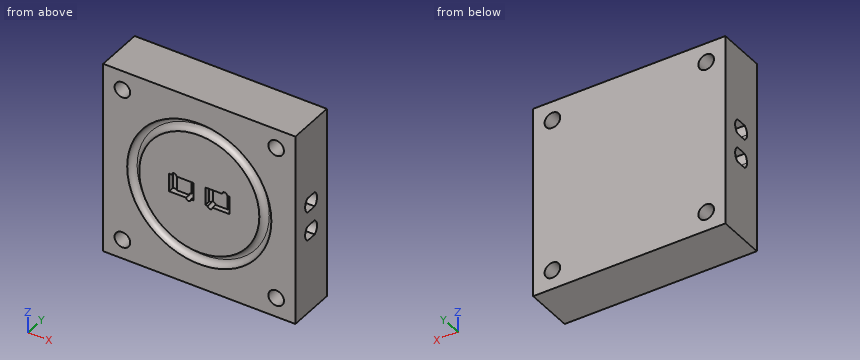
from build123d import *

# Parameters (mm, degrees)
F1_W      = 80
F1_H      = 80
F2_DEPTH  = 20
F4_R      = 3.25
F5_DEPTH  = 20.001
F4_R_2    = 30
F4_R_3    = 25
F6_DEPTH  = 2.5
F7_R      = 2.49999
F4_W      = 2
F4_H      = 3.75
F9_DEPTH  = 2.5
F10_DEPTH = 10
F12_DEPTH = 80.001
F13_DEPTH = 80.0010001
F14_DEPTH = 2


# Not quite as in the source:
# - two fillets or chamfers of one size are made in one step
# - a fillet or chamfer is up to 0.001 mm smaller than in the source, because OpenCascade refuses the exact size


with BuildPart() as f2:
    # F1 (on Front) → F2 (new body)
    with BuildSketch(Plane.XZ):
        with Locations((40, 40)):
            Rectangle(F1_W, F1_H)
    extrude(amount=F2_DEPTH)

    # F4 (on face) → F5 (cut, through all)
    with BuildSketch(Plane.XZ.offset(20)):
        with Locations((72, 8)):
            Circle(F4_R)
        with Locations((8, 8)):
            Circle(F4_R)
        with Locations((8, 72)):
            Circle(F4_R)
        with Locations((72, 72)):
            Circle(F4_R)
    extrude(amount=-F5_DEPTH, mode=Mode.SUBTRACT)

    # F4 (on face) → F6 (cut)
    with BuildSketch(Plane.XZ.offset(20)):
        with Locations((40, 40)):
            Circle(F4_R_2)
        with Locations((40, 40)):
            Circle(F4_R_3, mode=Mode.SUBTRACT)
    extrude(amount=-F6_DEPTH, mode=Mode.SUBTRACT)

    # F7 (radius 2.5 in the source; OpenCascade refuses exactly that, so slightly less here)
    f7_edges = [f2.edges().sort_by_distance(p)[0] for p in [
        (15, -17.5, 40),
        (10, -17.5, 40),
    ]]
    fillet(f7_edges, radius=F7_R)

    # F4 (on face) → F9 (cut)
    with BuildSketch(Plane.XZ.offset(20)):
        with BuildLine():
            Line((28.5, 43.75), (27.5, 43.75))
            Line((27.5, 43.75), (27.5, 40))
            Line((27.5, 40), (29.5, 40))
            Line((29.5, 40), (29.5, 42.75))
            ThreePointArc((29.5, 42.75), (28.7928932188, 43.0428932188), (28.5, 43.75))
        make_face()
        with Locations((28.5, 38.125)):
            Rectangle(F4_W, F4_H)
        with BuildLine():
            ThreePointArc((30.5, 43.75), (29.5, 44.75), (28.5, 43.75))
            Line((28.5, 43.75), (29.5, 43.75))
            Line((29.5, 43.75), (30.5, 43.75))
        make_face()
        with BuildLine():
            Line((52.5, 40), (52.5, 43.75))
            Line((52.5, 43.75), (51.5, 43.75))
            ThreePointArc((51.5, 43.75), (51.2071067812, 43.0428932188), (50.5, 42.75))
            Line((50.5, 42.75), (50.5, 40))
            Line((50.5, 40), (52.5, 40))
        make_face()
        with BuildLine():
            Line((37.5, 36.25), (37.5, 40))
            Line((37.5, 40), (35.5, 40))
            Line((35.5, 40), (35.5, 37.25))
            ThreePointArc((35.5, 37.25), (36.2071067812, 36.9571067812), (36.5, 36.25))
            Line((36.5, 36.25), (37.5, 36.25))
        make_face()
        with Locations((36.5, 41.875)):
            Rectangle(F4_W, F4_H)
        with Locations((43.5, 41.875)):
            Rectangle(F4_W, F4_H)
        with BuildLine():
            Line((44.5, 40), (42.5, 40))
            Line((42.5, 40), (42.5, 36.25))
            Line((42.5, 36.25), (43.5, 36.25))
            ThreePointArc((43.5, 36.25), (43.7928932188, 36.9571067812), (44.5, 37.25))
            Line((44.5, 37.25), (44.5, 40))
        make_face()
        with Locations((51.5, 38.125)):
            Rectangle(F4_W, F4_H)
        with BuildLine():
            Line((50.5, 43.75), (51.5, 43.75))
            ThreePointArc((51.5, 43.75), (50.5, 44.75), (49.5, 43.75))
            Line((49.5, 43.75), (50.5, 43.75))
        make_face()
        with BuildLine():
            ThreePointArc((36.5, 36.25), (36.2071067812, 36.9571067812), (35.5, 37.25))
            Line((35.5, 37.25), (35.5, 36.25))
            Line((35.5, 36.25), (36.5, 36.25))
        make_face()
        with BuildLine():
            Line((44.5, 36.25), (44.5, 37.25))
            ThreePointArc((44.5, 37.25), (43.7928932188, 36.9571067812), (43.5, 36.25))
            Line((43.5, 36.25), (44.5, 36.25))
        make_face()
    extrude(amount=-F9_DEPTH, mode=Mode.SUBTRACT)

    # F4 (on face) → F10 (cut)
    with BuildSketch(Plane.XZ.offset(20)):
        with BuildLine():
            ThreePointArc((30.5, 43.75), (29.5, 44.75), (28.5, 43.75))
            Line((28.5, 43.75), (29.5, 43.75))
            Line((29.5, 43.75), (30.5, 43.75))
        make_face()
        with BuildLine():
            Line((29.5, 43.75), (28.5, 43.75))
            ThreePointArc((28.5, 43.75), (28.7928932188, 43.0428932188), (29.5, 42.75))
            Line((29.5, 42.75), (29.5, 43.75))
        make_face()
        with BuildLine():
            Line((30.5, 43.75), (29.5, 43.75))
            Line((29.5, 43.75), (29.5, 42.75))
            ThreePointArc((29.5, 42.75), (30.2071067812, 43.0428932188), (30.5, 43.75))
        make_face()
        with BuildLine():
            Line((35.5, 36.25), (35.5, 37.25))
            ThreePointArc((35.5, 37.25), (34.7928932188, 36.9571067812), (34.5, 36.25))
            Line((34.5, 36.25), (35.5, 36.25))
        make_face()
        with BuildLine():
            ThreePointArc((36.5, 36.25), (36.2071067812, 36.9571067812), (35.5, 37.25))
            Line((35.5, 37.25), (35.5, 36.25))
            Line((35.5, 36.25), (36.5, 36.25))
        make_face()
        with BuildLine():
            ThreePointArc((34.5, 36.25), (35.5, 35.25), (36.5, 36.25))
            Line((36.5, 36.25), (35.5, 36.25))
            Line((35.5, 36.25), (34.5, 36.25))
        make_face()
        with BuildLine():
            Line((44.5, 36.25), (44.5, 37.25))
            ThreePointArc((44.5, 37.25), (43.7928932188, 36.9571067812), (43.5, 36.25))
            Line((43.5, 36.25), (44.5, 36.25))
        make_face()
        with BuildLine():
            ThreePointArc((45.5, 36.25), (45.2071067812, 36.9571067812), (44.5, 37.25))
            Line((44.5, 37.25), (44.5, 36.25))
            Line((44.5, 36.25), (45.5, 36.25))
        make_face()
        with BuildLine():
            Line((44.5, 36.25), (43.5, 36.25))
            ThreePointArc((43.5, 36.25), (44.5, 35.25), (45.5, 36.25))
            Line((45.5, 36.25), (44.5, 36.25))
        make_face()
        with BuildLine():
            Line((50.5, 43.75), (51.5, 43.75))
            ThreePointArc((51.5, 43.75), (50.5, 44.75), (49.5, 43.75))
            Line((49.5, 43.75), (50.5, 43.75))
        make_face()
        with BuildLine():
            Line((50.5, 42.75), (50.5, 43.75))
            Line((50.5, 43.75), (49.5, 43.75))
            ThreePointArc((49.5, 43.75), (49.7928932188, 43.0428932188), (50.5, 42.75))
        make_face()
        with BuildLine():
            ThreePointArc((50.5, 42.75), (51.2071067812, 43.0428932188), (51.5, 43.75))
            Line((51.5, 43.75), (50.5, 43.75))
            Line((50.5, 43.75), (50.5, 42.75))
        make_face()
    extrude(amount=-F10_DEPTH, mode=Mode.SUBTRACT)

    # F11 (on face) → F12 (cut, through all)
    with BuildSketch(Plane(origin=(0, 0, 0), x_dir=(0, -1, 0), z_dir=(-1, 0, 0))):
        with BuildLine():
            ThreePointArc((12.2666053913, 42.95), (13.3950773546, 44.293116947), (13.8, 46))
            ThreePointArc((13.8, 46), (13.3950773546, 47.706883053), (12.2666053913, 49.05))
            Line((12.2666053913, 49.05), (7.7333946087, 49.05))
            ThreePointArc((7.7333946087, 49.05), (6.2, 46), (7.7333946087, 42.95))
            Line((7.7333946087, 42.95), (12.2666053913, 42.95))
        make_face()
    extrude(amount=-F12_DEPTH, mode=Mode.SUBTRACT)

    # F11 (on face) → F13 (cut, through all)
    with BuildSketch(Plane(origin=(0, 0, 0), x_dir=(0, -1, 0), z_dir=(-1, 0, 0))):
        with BuildLine():
            ThreePointArc((12.2666053913, 42.95), (13.3950773546, 44.293116947), (13.8, 46))
            ThreePointArc((13.8, 46), (13.3950773546, 47.706883053), (12.2666053913, 49.05))
            Line((12.2666053913, 49.05), (7.7333946087, 49.05))
            ThreePointArc((7.7333946087, 49.05), (6.2, 46), (7.7333946087, 42.95))
            Line((7.7333946087, 42.95), (12.2666053913, 42.95))
        make_face()
        with BuildLine():
            ThreePointArc((12.2666053913, 30.95), (13.3950773546, 32.293116947), (13.8, 34))
            ThreePointArc((13.8, 34), (13.3950773546, 35.706883053), (12.2666053913, 37.05))
            Line((12.2666053913, 37.05), (7.7333946087, 37.05))
            ThreePointArc((7.7333946087, 37.05), (6.2, 34), (7.7333946087, 30.95))
            Line((7.7333946087, 30.95), (12.2666053913, 30.95))
        make_face()
    extrude(amount=-F13_DEPTH, mode=Mode.SUBTRACT)

    # F4 (on face) → F14 (cut)
    with BuildSketch(Plane.XZ.offset(20)):
        with BuildLine():
            Line((29.5, 42.75), (29.5, 40))
            Line((29.5, 40), (35.5, 40))
            Line((35.5, 40), (35.5, 43.75))
            Line((35.5, 43.75), (30.5, 43.75))
            ThreePointArc((30.5, 43.75), (30.2071067812, 43.0428932188), (29.5, 42.75))
        make_face()
        with BuildLine():
            Line((35.5, 40), (29.5, 40))
            Line((29.5, 40), (29.5, 36.25))
            Line((29.5, 36.25), (34.5, 36.25))
            ThreePointArc((34.5, 36.25), (34.7928932188, 36.9571067812), (35.5, 37.25))
            Line((35.5, 37.25), (35.5, 40))
        make_face()
        with BuildLine():
            Line((44.5, 43.75), (44.5, 40))
            Line((44.5, 40), (50.5, 40))
            Line((50.5, 40), (50.5, 42.75))
            ThreePointArc((50.5, 42.75), (49.7928932188, 43.0428932188), (49.5, 43.75))
            Line((49.5, 43.75), (44.5, 43.75))
        make_face()
        with BuildLine():
            Line((50.5, 40), (44.5, 40))
            Line((44.5, 40), (44.5, 37.25))
            ThreePointArc((44.5, 37.25), (45.2071067812, 36.9571067812), (45.5, 36.25))
            Line((45.5, 36.25), (50.5, 36.25))
            Line((50.5, 36.25), (50.5, 40))
        make_face()
    extrude(amount=-F14_DEPTH, mode=Mode.SUBTRACT)


solid = f2.part
Part model, mm, in its own coordinate system. Give positions to 0.01 mm unless a question says otherwise; leave off trailing zeros. Loops run counter-clockwise (first coordinate to the right, second up) from the corner with the lowest first, then second, coordinate; pieces in that order, holes last. Notation, with made-up numbers: M -8.5,-26 L -4.5,-26 A15 cw -4.5,-10 Z; hole C -36,82.5 d10. An arc over 180 degrees is marked long. Put each result on its own line as item: value. Start each with the question number.
1) Probe probe 1 along Z at (x, y) = (72, -8.5); probe 2 along Z at (x, y) = (32, -9.5); probe 3 along X at (y, z) = (-17.25, 43.75). List the from-to ranges inside material, lowest first.
2) Saw through at C-C (y = -4.75). List the corners of the cut face in (x, z).
3) Saw through at B-B (z = 72). List the corners of the cut face in (x, y), then the cut area to 3 significant figures.
4) Flat gauge pin, fed straight in: pin 1 (0.6 mm diameter, centred on x = 51, z = 39, fed in from -Y). Where does the tip first touch, or does it go through?
5) Saw through at A-A (x = 8). List the corners of the cut face in (y, z), then the cut area to 3 significant figures.
6) Saw through at D-D (x = 33). State how many separate pieces and enclosed holes the cut face has, then the cut area to 3 significant figures.
Numbers:
1. probe 1: 0 to 4.75, 11.25 to 30.95, 37.05 to 42.95, 49.05 to 68.75, 75.25 to 80
1. probe 2: 0 to 30.95, 37.05 to 42.95, 49.05 to 80
1. probe 3: 0 to 28.5, 30.5 to 49.5, 51.5 to 80
2. outline: M 0,0 L 80,0 L 80,80 L 0,80 Z; hole C 8,8 d6.5; hole C 8,72 d6.5; hole C 72,8 d6.5; hole C 72,72 d6.5
3. outline: M 0,-20 L 4.75,-20 L 4.75,0 L 0,0 Z; M 11.25,-20 L 68.75,-20 L 68.75,0 L 11.25,0 Z; M 75.25,-20 L 80,-20 L 80,0 L 75.25,0 Z
3. area: 1,340 mm^2
4. pin 1: y = -17.5
5. outline: M -20,0 L 0,0 L 0,4.75 L -20,4.75 Z; M -20,11.25 L 0,11.25 L 0,68.75 L -20,68.75 Z; M -20,75.25 L 0,75.25 L 0,80 L -20,80 Z; hole M -12.27,30.95 L -7.73,30.95 A3.8 ccw -7.73,37.05 L -12.27,37.05 A3.8 ccw Z; hole M -12.27,42.95 L -7.73,42.95 A3.8 ccw -7.73,49.05 L -12.27,49.05 A3.8 ccw Z
5. area: 1,260 mm^2
6. separate pieces: 1
6. enclosed holes: 2
6. area: 1,480 mm^2
